Could you check a few things on this drawing? It's one solid part, dimensions in mm from its lowest x, y, z. A direction names the side the tool comes from. Give positions to 0.01 mm unless a question says otherwise; leave off trailing zeros. Loops run counter-clockwise (first coordinate to the right, second up) from the corner with the lowest first, then second, coordinate; pieces in that order, holes last. Notation, with made-up numbers: M 67.25,60.5 L 119.25,60.5 A8 ccw 119.25,70.5 Z; hole C 4.25,-28 d2. An arc over 180 degrees is marked long. Answer in a Markdown table with one row per item. Add a question column.
1. If we section it at B-B on y = 11.5: List the corners of the cut face in (x, z) for me.
2. I'm going to push flat-ended pins straight in: pin 1 Ø10 at (x, y) = (16.5, 13) entering from +Z; pin 2 Ø10 at (x, z) = (22.5, 20.5) entering from -Y; pin 3 Ø2.5 at (y, z) = (22, 11) entering from +X. Where does each tip first touch, or does it pass through?
3. Which directions (+Z, -Z, +X, -X, +Y, -Y) give clear straight access to the entire face, cutting with the end or side of a thin tool? Please do the marked faces 1 and 2.
4. If we section it at A-A on x = 19: List the corners of the cut face in (y, z) for me.
5. If we section it at D-D on z = 22: List the corners of the cut face in (x, y) for me, then the cut area to 3 significant figures.
6. If we section it at C-C on y = 21.5: List the corners of the cut face in (x, z) for me, then the cut area to 3 significant figures.
7. I need wall thicknesses on line 1 along X through (y, z) = (11.5, 0.8); line 2 along Z through (x, y) = (9, 21.4); line 3 along Y through (x, z) = (19, 0.7). Which ranges of each line are inside material? Lowest first, please. Write a range as from..to.
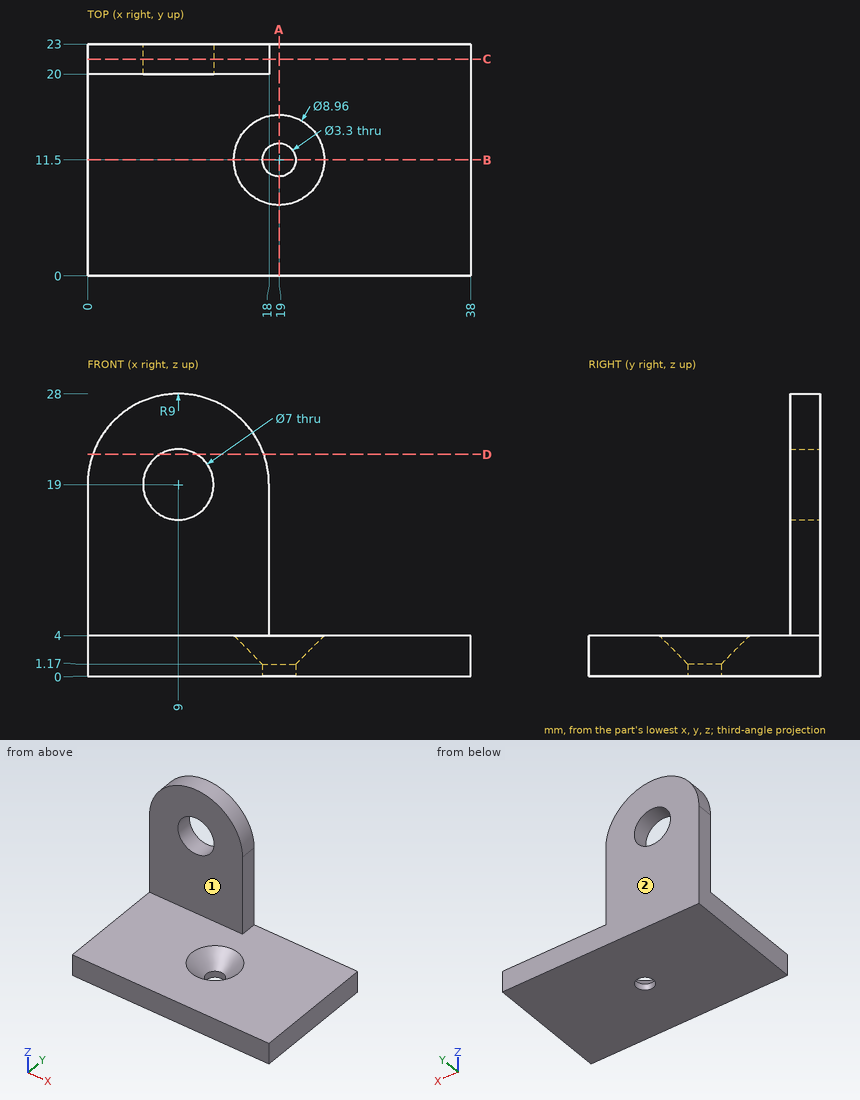
Results:
| question | item | result |
|---|---|---|
| 1 | outline | M 0,0 L 17.35,0 L 17.35,1.17 L 14.52,4 L 0,4 Z; M 20.65,0 L 38,0 L 38,4 L 23.48,4 L 20.65,1.17 Z |
| 2 | pin 1 | z = 4 |
| 2 | pin 2 | y = 20 |
| 2 | pin 3 | x = 18 |
| 3 | face 1 | +Z, +X, -X, -Y |
| 3 | face 2 | +Z, -Z, +X, -X, +Y |
| 4 | outline | M 0,0 L 9.85,0 L 9.85,1.17 L 7.02,4 L 0,4 Z; M 13.15,0 L 23,0 L 23,4 L 15.98,4 L 13.15,1.17 Z |
| 5 | outline | M 0.51,20 L 7.2,20 L 7.2,23 L 0.51,23 Z; M 10.8,20 L 17.49,20 L 17.49,23 L 10.8,23 Z |
| 5 | area | 40.1 mm2 |
| 6 | outline | M 0,0 L 38,0 L 38,4 L 18,4 L 18,19 A9 ccw 0,19 Z; hole C 9,19 d7 |
| 6 | area | 511 mm2 |
| 7 | line 1 | 0..17.35, 20.65..38 |
| 7 | line 2 | 0..15.5, 22.5..28 |
| 7 | line 3 | 0..9.85, 13.15..23 |
